The model under review builds one solid part; all positions refer to its coordinate system, in mm. A direction names the side the tool comes from. Round coordinates to 2 decimals unless told otherwise and drop trailing zeros. Order: outer loops, then holes, each group sorted by start corner. A loop starts at its lowest first (then second) coordinate and runs counter-clockwise, first axis right, second up. Notation, with made-up numbers: M 32,14.5 L 51,14.5 A11 cw 51,27.5 Z; hole C -39.5,-40 d7. An arc over 180 degrees is marked long. Use a Markdown table: item, result. Add a question column.
1. To check wall thickness, follow probe 1 along Y at (x, z) = (-10.75, -3.5); probe 2 along X at (y, z) = (0, 10.25); probe 3 along X at (y, z) = (0.25, -1.25). State the ranges of each line that lie inside material, in increasing order.
2. Insertion check: P1, Ø2, axis at x = -6.5, y = 4, coming from the -Z side; P2, Ø6, axis at y = 1, z = 8.5, coming from the +X side; P3, Ø3, axis at x = -12.5, z = -1.5, coming from the -Y side; P4, Ø6, axis at y = -5, z = 4.5, coming from the -X side. Each pin has a flat end and moves straight along its axis. Give the tip position at first contact, or say it passes through.
3. Consider section A-A on z = -1.25. State the section outline as (x, y) points.
4. The part is to be moulded in two halves that separate along Y. For faces 3 (the conical face through (-11.7, -0.08, 10.15)), 4 (the flat face through (-11.2, 1.5, -7.747)), 5 (the cylindrical face through (-5.91, -4.64, -0.84)), say which applies: +Y half, -Y half, draft (parallel to the pull), parting line (faces both ways), or undercut.
5. Consider section C-C on z = 4.75. State the section outline as (x, y) points.
6. For faces 1 (the cylindrical face through (-14.985, 0.954, -4.656)), 2 (the conical face through (-9.563, -1.836, 9.897)), list the 3-axis set-ups (+Z, -Z, +X, -X, +Y, -Y) from which the entire face can be reached by the end or side of a thin tool; tool diameter is ignored.
7. Consider section B-B on z = 14.75. State the section outline as (x, y) points.
from build123d import *

# Parameters (mm, degrees)
F0_W     = 3.175
F0_H     = 6.096
F3_D     = 3.048
F3_DEPTH = 17.145
F3_TIP   = 0.9157115834


with BuildPart() as f1:
    # F0 (on Front) → F1 (revolve)
    with BuildSketch(Plane.XZ):
        Polygon((-11.9569151578, -1.651), (-11.9569151578, 16.383), (-19.5769151578, 0), (-19.5769151578, -1.651), (-15.1319151578, -1.651), align=None)
        with Locations((-13.5444151578, -4.699)):
            Rectangle(F0_W, F0_H)
    revolve(axis=Axis((-11.9569151578, 0, 7.366), (0, 0, -1)))

    # F3
    with Locations(Plane(origin=(0, 0, -7.747), x_dir=(1, 0, 0), z_dir=(0, 0, -1))):
        with Locations((-11.9569151578, 0)):
            Hole(F3_D / 2, depth=F3_DEPTH)
            with Locations((0, 0, -(F3_DEPTH + F3_TIP / 2))):  # 118° drill point
                Cone(0, F3_D / 2, F3_TIP, mode=Mode.SUBTRACT)


solid = f1.part
Answer block:
| question | item | result |
|---|---|---|
| 1 | probe 1 | -2.94 to -0.93, 0.93 to 2.94 |
| 1 | probe 2 | -14.81 to -12.06, -11.85 to -9.1 |
| 1 | probe 3 | -19.57 to -13.46, -10.45 to -4.34 |
| 2 | P1 | z = -1.65 |
| 2 | P2 | x = -6.94 |
| 2 | P3 | y = -7.62 |
| 2 | P4 | x = -17.8 |
| 3 | outline | C -11.96,0 d15.24; hole C -11.96,0 d3.05 |
| 4 | face 3 | undercut |
| 4 | face 4 | draft |
| 4 | face 5 | parting line |
| 5 | outline | C -11.96,0 d10.82; hole C -11.96,0 d3.05 |
| 6 | face 1 | -Z |
| 6 | face 2 | +Z |
| 7 | outline | C -11.96,0 d1.52 |
